The listing builds one solid part. Answer for the finished solid, in the listing's coordinates (mm). A direction names the side the tool comes from. Round coordinates to 2 decimals unless told otherwise and drop trailing zeros. Write each loop counter-clockwise with the first axis right and the second up, starting at its lowest first coordinate (ties: lowest second). Pieces come first, ordered by that corner, then holes.
(1) Find the intervals of material crossed by probe 1 along X at (y, z) = (9.5, 0); probe 2 along Z at (x, y) = (-1, 9.75); probe 3 along Y at (x, z) = (6.5, -2.25), in increasing order.
(2) A cutting plane is placed at C-C, the plane y = 2.25. Give the vertices of the cut face in (x, z), and give its area (3 significant figures).
(3) A cutting plane is placed at D-D, the plane z = -4.75. Give the vertices of the cut face in (x, y).
(4) Each of these flat-tipped pins is pushed along its axis until it touches: pin 1 Ø6 at (y, z) = (3.5, 3.5) entering from +X; pin 2 Ø8 at (x, z) = (2, 3.5) entering from -Y; pin 3 Ø1.2 at (x, z) = (0, -4) entering from +Y; pin 4 Ø4 at (x, y) = (-1.5, 1.5) entering from -Z. Where does it stop, or does it pass through?
(5) A cutting plane is placed at A-A, the plane z = 0. Give the vertices of the cut face in (x, y).
(6) The mould has two halves that part along X. Classify faces 4 (the face through (0, 2.5, -5)), 5 (the face through (0, 12.5, 2)), 6 (the face through (-1.802, 3.698, -5.723)), 7 (the face through (0.05, 7.57, -5.75)): +X half, -X half, draft (parallel to the pull), parting line (faces both ways), or undercut.
(7) A cutting plane is placed at B-B, the plane x = 0. Give the vertices of the cut face in (y, z).
(8) For faces 1 (the face through (-1.4, 0, 0.1)), 2 (the face through (5, 7.5, -4)), 3 (the face through (0, 2.5, 5)), determine the directions among +Z, -Z, +X, -X, +Y, -Y from which every point of the face is accessible in a straight line to the end or side of a thin tool.
from build123d import *

# Parameters (mm, degrees)
ESQUISSE2_R             = 1.25
ENL_V_MAT_EXTRU_1_DEPTH = 10


with BuildPart() as part:
    # Esquisse1 → Révolution1 (revolve)
    with BuildSketch(Plane.XY, mode=Mode.PRIVATE) as r_volution1_sk:
        Polygon((7.75, 12.5), (7.75, 7.5), (6, 7.5), (6, 0), (1.25, 0), (1.25, 12.5), align=None)
    revolve(r_volution1_sk.sketch.rotate(Axis((0, 0, 0), (0, 1, 0)), 90), axis=Axis((0, 0, 0), (0, 1, 0)))

    # Esquisse2 → Enlèv. mat.-Extru.1 (cut)
    with BuildSketch(Plane(origin=(0, 12.5, 0), x_dir=(1, 0, 0), z_dir=(0, 1, 0))):
        with Locations(Location((0, 4.5, 0), (0, 0, 270))):
            Circle(ESQUISSE2_R)
        with Locations(Location((0, -4.5, 0), (0, 0, 90))):
            Circle(ESQUISSE2_R)
    extrude(amount=-ENL_V_MAT_EXTRU_1_DEPTH, mode=Mode.SUBTRACT)


solid = part.part
Solutions:
1. probe 1: x = -7.75 to -1.25, 1.25 to 7.75
1. probe 2: z = -7.69 to -5.25, -3.75 to -0.75, 0.75 to 3.75, 5.25 to 7.69
1. probe 3: y = 7.5 to 12.5
2. outline: circle Ø12 at (0, 0); hole circle Ø2.5 at (0, 0)
2. area: 108 mm2
3. outline: (-6.12, 7.5) - (-3.67, 7.5) - (-3.67, 0) - (3.67, 0) - (3.67, 7.5) - (6.12, 7.5) - (6.12, 12.5) - (1.22, 12.5) - (1.22, 2.5) - (-1.22, 2.5) - (-1.22, 12.5) - (-6.12, 12.5) - close
4. pin 1: stops at x = 5.98
4. pin 2: stops at y = 0
4. pin 3: stops at y = 2.5
4. pin 4: stops at z = -6
5. outline: (-7.75, 7.5) - (-6, 7.5) - (-6, 0) - (-1.25, 0) - (-1.25, 12.5) - (-7.75, 12.5) - close; (1.25, 0) - (6, 0) - (6, 7.5) - (7.75, 7.5) - (7.75, 12.5) - (1.25, 12.5) - close
6. face 4: undercut
6. face 5: draft
6. face 6: parting line
6. face 7: undercut
7. outline: (0, -6) - (7.5, -6) - (7.5, -7.75) - (12.5, -7.75) - (12.5, -5.75) - (2.5, -5.75) - (2.5, -3.25) - (12.5, -3.25) - (12.5, -1.25) - (0, -1.25) - close; (0, 1.25) - (12.5, 1.25) - (12.5, 3.25) - (2.5, 3.25) - (2.5, 5.75) - (12.5, 5.75) - (12.5, 7.75) - (7.5, 7.75) - (7.5, 6) - (0, 6) - close
8. face 1: +Z, -Z, +X, -X, -Y
8. face 2: -Y
8. face 3: +Y
